The model under review builds one solid part; all positions refer to its coordinate system, in mm. A direction names the side the tool comes from. Coordinates: 2 decimals unless noted, no trailing zeros. Loops run counter-clockwise (first coordinate to the right, second up) from the corner with the lowest first, then second, coordinate; pieces in that order, holes last. Notation, with made-up numbers: M 25,-7 L 83,-7 A20 cw 83,0 Z; hole C -9.75,25.25 d8. An arc over 180 degrees is marked long. One line per item, written item: value.
Autodesk Inventor part; units mm, degrees
ref_plane "Arbeitsebene1" through (0, -16, 0) normal (0, 1, 0) x (-1, 0, 0)
ref_plane "YZ Plane" through (0, 0, 0) normal (1, 0, 0) x (0, 1, 0)
ref_plane "XY Plane" through (0, 0, 0) normal (0, 0, 1) x (1, 0, 0)
sketch "Skizze1" plane through (0, 0, 0) normal (0, 1, 0) x (-1, 0, 0)
  line L0 (-15, 16) -> (-7.5, 16)
  line L1 (-7.5, 16) -> (-7.5, -10)
  line L2 (-15, 16) -> (-15, 6)
  line L3 (-15, 6) -> (-35, 6)
  line L4 (-35, 6) -> (-35, 0)
  line L5 (-35, 0) -> (-15, 0)
  line L6 (-15, 0) -> (-15, -10)
  line L7 (0, -15.2) -> (0, 21.2)
  line L8 (-7.5, -10) -> (-15, -10)
  point P0 (0, 0)
  dimension "d0" = 30
  dimension "d1" = 15
  dimension "d2" = 70
  dimension "d3" = 6
  dimension "d4" = 10
  dimension "d5" = 10
revolve "Umdrehung1" add sketch "Skizze1" angle 360 about axis through (0, 0, -10) along (0, 0, 1)
ref_plane "Arbeitsebene1" through (0, -16, 0) normal (0, 1, 0) x (-1, 0, 0)
sketch "Skizze2" plane through (0, -16, 0) normal (0, 1, 0) x (-1, 0, 0)
  line L0 (15, 16) -> (-15, 16)
  line L1 (15, 6) -> (-15, 6)
  line L2 (6, 16) -> (-6, 16)
  line L3 (-6, 16) -> (-6, 6)
  line L4 (-6, 6) -> (6, 6)
  line L5 (6, 6) -> (6, 16)
  line L6 (0, -2.8) -> (0, 16.8)
  point P0 (0, 0)
  dimension "d8" = 12
extrude "Extrusion1" cut sketch "Skizze2" along normal blind 2
sketch "Skizze4" plane through (0, -14, 0) normal (0, -1, 0) x (1, 0, 0)
  line L0 (-5.3852, 16) -> (5.3852, 16)
  point P0 (0, 0)
  point P1 (-0.0015, 10)
  dimension "d18" = 6
hole "Bohrung2" at (-0.0015, -14, 10) direction (0, 1, 0) diameter 3.3 depth 10 tip angle 118
thread "Gewinde1"
sketch "Skizze6" plane through (0, 0, 6) normal (0, 0, 1) x (1, 0, 0)
  circle A0 centre (0, 0) radius 35
  point P0 (0, 26)
  point P1 (-22.5167, -13)
  point P2 (22.5167, -13)
  dimension "d40" = 26
  dimension "d41" = 0
  dimension "d44" = 360
hole "Bohrung4" at (0, 26, 6) at (-22.5167, -13, 6) at (22.5167, -13, 6) direction (0, 0, -1) diameter 6.5 depth 35 tip angle 118
chamfer "Fase1" distance 1 angle 45 1 edges at (-15, 0, -10)
properties part number "Matrizenhalterung_unten" material "Stahl"
(1) Add section D-D on y = 26. State the section outline as (x, z) points.
Checks:
outline: M -23.43,0 L -3.25,0 L -3.25,6 L -23.43,6 Z; M 3.25,0 L 23.43,0 L 23.43,6 L 3.25,6 Z
(2) Add section C-C on y = -13. State how many separate pieces and enclosed holes the cut face has, then the cut area to 3 significant figures.
Checks:
separate pieces: 3
enclosed holes: 1
area: 601 mm^2
(3) Add section A-A on y = 0. State the section outline as (x, z) points.
Checks:
outline: M -35,0 L -15,0 L -15,-9 L -14,-10 L -7.5,-10 L -7.5,16 L -15,16 L -15,6 L -35,6 Z; M 7.5,-10 L 14,-10 L 15,-9 L 15,0 L 35,0 L 35,6 L 15,6 L 15,16 L 7.5,16 Z
(4) To check wall thickness, follow L1, parallel to Y at x = 0, z = 2.7; L2, parallel to X at y = -13, z = 2.35; L3, parallel to Z at x = 20, y = 19. State the ranges of each line that lie inside material, in increasing order. Write a range as [from, to].
Checks:
L1: [-35, -7.5], [7.5, 22.75], [29.25, 35]
L2: [-32.5, -25.77], [-19.27, 19.27], [25.77, 32.5]
L3: [0, 6]
(5) Insertion check: pin 1 Ø19.5 at (x, y) = (0, 0) entering from +Z; pin 2 Ø6 at (x, z) = (-11.5, -2) entering from +Y; pin 3 Ø10 at (y, z) = (-16, 9) entering from +X; pin 4 Ø8 at (y, z) = (23.5, 9) entering from +X. Each pin has a flat end and moves straight along its axis. Give the tip position at first contact, or say it passes through.
Checks:
pin 1: z = 16
pin 2: y = 33.75
pin 3: x = 32.88
pin 4: x = 28.11
(6) Draft analysis for pull direction Z (two halves, no side actions). For faces 5 (the face through (6, -6, -10)), 6 (the face through (3.1, 7.1, 16)), 7 (the face through (0.63, -10.611, 8.476)), 8 (the face through (-0.98, 22.9, 2.96)), state which applies: pulls with the +Z half, pulls with the -Z half, needs draft (parallel to the pull), parting line crosses it, or undercut.
Checks:
face 5: pulls with the -Z half
face 6: pulls with the +Z half
face 7: undercut
face 8: needs draft
(7) Tool access review of faces 1 (the face through (-0.58, 14.99, 10.93)), 2 (the face through (-22.66, -9.753, 2.958)), 3 (the face through (0, -14, 12)), 4 (the face through (15, -7, 0)): name each direction out of +Z, -Z, +X, -X, +Y, -Y from which nothing blocks a thin tool from reaching the whole face with its end or side.
Checks:
face 1: +Z
face 2: +Z, -Z
face 3: +Z, +X, -X, -Y
face 4: -Z
(8) Add section B-B on z = -6.75. State the section outline as (x, y) points.
Checks:
outline: C 0,0 d30; hole C 0,0 d15
